Autodesk Inventor part; units mm, degrees
ref_plane "YZ Plane" through (0, 0, 0) normal (1, 0, 0) x (0, 1, 0)
ref_plane "XZ Plane" through (0, 0, 0) normal (0, 1, 0) x (-1, 0, 0)
ref_plane "XY Plane" through (0, 0, 0) normal (0, 0, 1) x (1, 0, 0)
sketch "Sketch_1" plane through (0, 0, 0) normal (0, 0, 1) x (1, 0, 0)
  arc A0 (-12.6998, -10.5664) -> (-10.5664, -12.6998) centre (-10.5918, -10.5918) ccw
  arc A1 (-9.5504, -12.7) -> (-10.5664, -12.6998) centre (-10.0584, -12.7) ccw
  line L0 (-9.5504, -12.7) -> (-6.3331, -12.7)
  arc A2 (-5.3171, -12.7) -> (-6.3331, -12.7) centre (-5.8251, -12.7) ccw
  line L1 (-5.3171, -12.7) -> (-4.3434, -12.7)
  arc A3 (-4.3434, -12.7) -> (-4.3434, -10.4902) centre (-4.3434, -11.5951) ccw
  line L2 (-4.3434, -10.4902) -> (-6.4748, -10.4902)
  arc A4 (-7.1932, -8.7558) -> (-6.4748, -10.4902) centre (-6.4748, -9.4742) ccw
  line L3 (-7.1932, -8.7558) -> (-3.8632, -5.4257)
  arc A5 (-1.6181, -4.4958) -> (-3.8632, -5.4257) centre (-1.6181, -7.6708) ccw
  line L4 (-1.6181, -4.4958) -> (1.6181, -4.4958)
  arc A6 (3.8632, -5.4257) -> (1.6181, -4.4958) centre (1.6181, -7.6708) ccw
  line L5 (3.8632, -5.4257) -> (7.1932, -8.7558)
  arc A7 (6.4748, -10.4902) -> (7.1932, -8.7558) centre (6.4748, -9.4742) ccw
  line L6 (6.4748, -10.4902) -> (4.3434, -10.4902)
  arc A8 (4.3434, -10.4902) -> (4.3434, -12.7) centre (4.3434, -11.5951) ccw
  line L7 (4.3434, -12.7) -> (5.3171, -12.7)
  arc A9 (6.3331, -12.7) -> (5.3171, -12.7) centre (5.8251, -12.7) ccw
  line L8 (6.3331, -12.7) -> (9.5504, -12.7)
  arc A10 (10.5664, -12.6998) -> (9.5504, -12.7) centre (10.0584, -12.7) ccw
  arc A11 (10.5664, -12.6998) -> (12.6998, -10.5664) centre (10.5918, -10.5918) ccw
  arc A12 (12.7, -9.5504) -> (12.6998, -10.5664) centre (12.7, -10.0584) ccw
  line L9 (12.7, -9.5504) -> (12.7, -6.3331)
  arc A13 (12.7, -5.3171) -> (12.7, -6.3331) centre (12.7, -5.8251) ccw
  line L10 (12.7, -5.3171) -> (12.7, -4.3434)
  arc A14 (12.7, -4.3434) -> (10.4902, -4.3434) centre (11.5951, -4.3434) ccw
  line L11 (10.4902, -4.3434) -> (10.4902, -6.4748)
  arc A15 (8.7558, -7.1932) -> (10.4902, -6.4748) centre (9.4742, -6.4748) ccw
  line L12 (8.7558, -7.1932) -> (5.4257, -3.8632)
  arc A16 (4.4958, -1.6181) -> (5.4257, -3.8632) centre (7.6708, -1.6181) ccw
  line L13 (4.4958, -1.6181) -> (4.4958, 1.6181)
  arc A17 (5.4257, 3.8632) -> (4.4958, 1.6181) centre (7.6708, 1.6181) ccw
  line L14 (5.4257, 3.8632) -> (8.7558, 7.1932)
  arc A18 (10.4902, 6.4748) -> (8.7558, 7.1932) centre (9.4742, 6.4748) ccw
  line L15 (10.4902, 6.4748) -> (10.4902, 4.3434)
  arc A19 (10.4902, 4.3434) -> (12.7, 4.3434) centre (11.5951, 4.3434) ccw
  line L16 (12.7, 4.3434) -> (12.7, 5.3171)
  arc A20 (12.7, 6.3331) -> (12.7, 5.3171) centre (12.7, 5.8251) ccw
  line L17 (12.7, 6.3331) -> (12.7, 9.5504)
  arc A21 (12.6998, 10.5664) -> (12.7, 9.5504) centre (12.7, 10.0584) ccw
  arc A22 (12.6998, 10.5664) -> (10.5664, 12.6998) centre (10.5918, 10.5918) ccw
  arc A23 (9.5504, 12.7) -> (10.5664, 12.6998) centre (10.0584, 12.7) ccw
  line L18 (9.5504, 12.7) -> (6.3331, 12.7)
  arc A24 (5.3171, 12.7) -> (6.3331, 12.7) centre (5.8251, 12.7) ccw
  line L19 (5.3171, 12.7) -> (4.3434, 12.7)
  arc A25 (4.3434, 12.7) -> (4.3434, 10.4902) centre (4.3434, 11.5951) ccw
  line L20 (4.3434, 10.4902) -> (6.4748, 10.4902)
  arc A26 (7.1932, 8.7558) -> (6.4748, 10.4902) centre (6.4748, 9.4742) ccw
  line L21 (7.1932, 8.7558) -> (3.8632, 5.4257)
  arc A27 (1.6181, 4.4958) -> (3.8632, 5.4257) centre (1.6181, 7.6708) ccw
  line L22 (1.6181, 4.4958) -> (-1.6181, 4.4958)
  arc A28 (-3.8632, 5.4257) -> (-1.6181, 4.4958) centre (-1.6181, 7.6708) ccw
  line L23 (-3.8632, 5.4257) -> (-7.1932, 8.7558)
  arc A29 (-6.4748, 10.4902) -> (-7.1932, 8.7558) centre (-6.4748, 9.4742) ccw
  line L24 (-6.4748, 10.4902) -> (-4.3434, 10.4902)
  arc A30 (-4.3434, 10.4902) -> (-4.3434, 12.7) centre (-4.3434, 11.5951) ccw
  line L25 (-4.3434, 12.7) -> (-5.3171, 12.7)
  arc A31 (-6.3331, 12.7) -> (-5.3171, 12.7) centre (-5.8251, 12.7) ccw
  line L26 (-6.3331, 12.7) -> (-9.5504, 12.7)
  arc A32 (-10.5664, 12.6998) -> (-9.5504, 12.7) centre (-10.0584, 12.7) ccw
  arc A33 (-10.5664, 12.6998) -> (-12.6998, 10.5664) centre (-10.5918, 10.5918) ccw
  arc A34 (-12.7, 9.5504) -> (-12.6998, 10.5664) centre (-12.7, 10.0584) ccw
  line L27 (-12.7, 9.5504) -> (-12.7, 6.3331)
  arc A35 (-12.7, 5.3171) -> (-12.7, 6.3331) centre (-12.7, 5.8251) ccw
  line L28 (-12.7, 5.3171) -> (-12.7, 4.3434)
  arc A36 (-12.7, 4.3434) -> (-10.4902, 4.3434) centre (-11.5951, 4.3434) ccw
  line L29 (-10.4902, 4.3434) -> (-10.4902, 6.4748)
  arc A37 (-8.7558, 7.1932) -> (-10.4902, 6.4748) centre (-9.4742, 6.4748) ccw
  line L30 (-8.7558, 7.1932) -> (-5.4257, 3.8632)
  arc A38 (-4.4958, 1.6181) -> (-5.4257, 3.8632) centre (-7.6708, 1.6181) ccw
  line L31 (-4.4958, 1.6181) -> (-4.4958, -1.6181)
  arc A39 (-5.4257, -3.8632) -> (-4.4958, -1.6181) centre (-7.6708, -1.6181) ccw
  line L32 (-5.4257, -3.8632) -> (-8.7558, -7.1932)
  arc A40 (-10.4902, -6.4748) -> (-8.7558, -7.1932) centre (-9.4742, -6.4748) ccw
  line L33 (-10.4902, -6.4748) -> (-10.4902, -4.3434)
  arc A41 (-10.4902, -4.3434) -> (-12.7, -4.3434) centre (-11.5951, -4.3434) ccw
  line L34 (-12.7, -4.3434) -> (-12.7, -5.3171)
  arc A42 (-12.7, -6.3331) -> (-12.7, -5.3171) centre (-12.7, -5.8251) ccw
  line L35 (-12.7, -6.3331) -> (-12.7, -9.5504)
  arc A43 (-12.6998, -10.5664) -> (-12.7, -9.5504) centre (-12.7, -10.0584) ccw
  circle A44 centre (0, 0) radius 2.6035
extrude "Extrusion1" add sketch "Sketch_1" against normal blind 38.1
properties part number "1010-15-CL"
CAD build for the part. Positions are in the model's coordinates, mm. A direction names the side the tool comes from. Round coordinates to 2 decimals unless told otherwise and drop trailing zeros. Order: outer loops, then holes, each group sorted by start corner. A loop starts at its lowest first (then second) coordinate and runs counter-clockwise, first axis right, second up. Notation, with made-up numbers: (71.25, 39.25) -> (89.25, 39.25) arc R17 cw to (89.25, 58.25) -> close; hole circle Ø11 at (-8, 50). An arc over 180 degrees is marked (long way). One line per question, with ' | ' between items.
Q1. Which spindle directions (+Z, -Z, +X, -X, +Y, -Y) get a long thin tool onto all of the face, cutting with end or side? Do faces 1 (the cylindrical face through (12.192, 5.836, -18.783)), 2 (the cylindrical face through (-3.24, 11.57, -18.78)). Say none if no direction does.
Completed:
face 1: +Z, -Z, +X | face 2: +Z, -Z
Q2. Probe probe 1 along Y at (x, z) = (0, -25.5); probe 2 along Y at (x, z) = (-6.75, -20); probe 3 along X at (y, z) = (-7, -36). List the from-to ranges inside material, lowest first.
Completed:
probe 1: y = -4.5 to -2.6, 2.6 to 4.5 | probe 2: y = -12.7 to -10.45, -8.31 to -5.19, 5.19 to 8.31, 10.45 to 12.7 | probe 3: x = -12.7 to -10.34, -8.56 to -5.44, 5.44 to 8.56, 10.34 to 12.7
Q3. Two-plate mould, pull along X, no slides. Class faces 3 (the flat face through (12.7, -8, -19)), 4 (the flat face through (0, -4.496, -19)), 5 (the flat face through (-12.7, 8, -19)): released by +X, released by -X, zero draft, split by the parting line, or undercut.
Completed:
face 3: released by +X | face 4: undercut | face 5: released by -X
Q4. Drop flat-ended pins along their axis: pin 1 (10 mm diameter, centred on y = 1.5, z = -9, fed in from -X); pin 2 (3.5 mm diameter, centred on y = 0, z = -24, fed in from -X); pin 3 (1 mm diameter, centred on y = -0.5, z = -24, fed in from +X); pin 4 (2.5 mm diameter, centred on x = 0, z = -22.5, fed in from -Y). Give the stop position or say it passes through.
Completed:
pin 1: stops at x = -12.7 | pin 2: stops at x = -4.5 | pin 3: stops at x = 4.5 | pin 4: stops at y = -4.5
Q5. Slice it at A-A (y = 0). Write the cut outline in (x, z), then the cut area to 3 significant figures.
Completed:
outline: (-4.5, -38.1) -> (-2.6, -38.1) -> (-2.6, 0) -> (-4.5, 0) -> close; (2.6, -38.1) -> (4.5, -38.1) -> (4.5, 0) -> (2.6, 0) -> close | area: 144 mm^2
